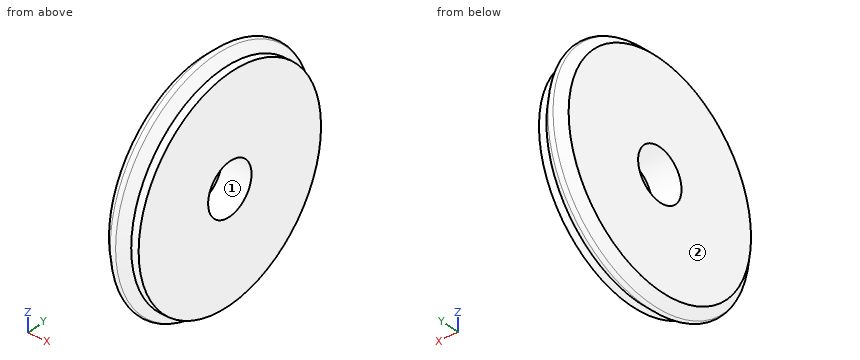
```python
from build123d import *

# Parameters (mm, degrees)
ESQUISSE6_W = 4
ESQUISSE6_H = 3.5


with BuildPart() as part:
    # Esquisse1 → Révolution1 (revolve)
    with BuildSketch(Plane.XY, mode=Mode.PRIVATE) as r_volution1_sk:
        with BuildLine():
            Line((0, 0), (0, 14.707106781))
            Line((0, 14.707106781), (1.146446609, 15.853553391))
            ThreePointArc((1.146446609, 15.853553391), (1.5, 16), (1.853553391, 15.853553391))
            Line((1.853553391, 15.853553391), (3, 14.707106781))
            Line((3, 14.707106781), (4, 14.707106781))
            Line((4, 14.707106781), (4, 0))
            Line((4, 0), (0, 0))
        make_face()
    revolve(r_volution1_sk.sketch.rotate(Axis((0, 0, 0), (1, 0, 0)), 180), axis=Axis((0, 0, 0), (1, 0, 0)))

    # Esquisse6 → Enlèvement de matière-Révolution1 (revolve, cut)
    with BuildSketch(Plane.XY, mode=Mode.PRIVATE) as enl_vement_de_mati_re_r_volution1_sk:
        with Locations((2, 1.75)):
            Rectangle(ESQUISSE6_W, ESQUISSE6_H)
    revolve(enl_vement_de_mati_re_r_volution1_sk.sketch.rotate(Axis((4, 0, 0), (-1, 0, 0)), 90), axis=Axis((4, 0, 0), (-1, 0, 0)), mode=Mode.SUBTRACT)


solid = part.part
```
Can you work these out from the model? Positions are in its coordinate system, mm. Face numbers are marked on the shaded views. Coordinates: 2 decimals unless noted, no trailing zeros. Loops run counter-clockwise (first coordinate to the right, second up) from the corner with the lowest first, then second, coordinate; pieces in that order, holes last. Notation, with made-up numbers: (-39, -2) -> (-11, -2) arc R16 cw to (-11, 16) -> close; hole circle Ø3 at (-20.5, 50.5). An arc over 180 degrees is marked (long way). Put each result on its own line as item: value. Start each with the question number.
Q1. If I drill on line 1 (Y direction, x = 0.95, z = -2); line 2 (Y direction, x = 2.75, z = 2.5); line 3 (Z direction, x = 1.75, y = 2), over which ranges is the centre line in solid material (lowest first)? Write a range as [from, to].
Q2. I'm going to push flat-ended pins straight in: P1, Ø1.5, axis at x = 2, z = 12.5, coming from the +Y side; P2, Ø1.5, axis at x = 1.5, z = -10, coming from the +Y side; P3, Ø4, axis at y = 0, z = 0, coming from the -X side. Where does each tip first touch, or does it pass through?
Q3. I want a section at A-A (y = 0). Write out the boundary of the cut face in (x, z).
Q4. Thinking about a two-plate mould opening in Y: for the marked faces 1 and 2, which applies, pulls with the +Y half, pulls with the -Y half, needs draft (parallel to the pull), parting line crosses it, or undercut?
Taken from the geometry:
1. line 1: y = [-15.53, -2.87], [2.87, 15.53]
1. line 2: y = [-14.75, -2.45], [2.45, 14.75]
1. line 3: z = [-15.81, -2.87], [2.87, 15.81]
2. P1: stops at y = 10.73
2. P2: stops at y = 13.06
2. P3: passes through
3. outline: (0, -14.71) -> (1.15, -15.85) arc R0.5 ccw to (1.85, -15.85) -> (3, -14.71) -> (4, -14.71) -> (4, -3.5) -> (0, -3.5) -> close; (0, 3.5) -> (4, 3.5) -> (4, 14.71) -> (3, 14.71) -> (1.85, 15.85) arc R0.5 ccw to (1.15, 15.85) -> (0, 14.71) -> close
4. face 1: undercut
4. face 2: needs draft
